Geometry: final body of the model. Coordinates: model frame, mm. Face numbers are marked on the shaded views. A direction names the side the tool comes from. Coordinates: 2 decimals unless noted, no trailing zeros. Loops run counter-clockwise (first coordinate to the right, second up) from the corner with the lowest first, then second, coordinate; pieces in that order, holes last. Notation, with made-up numbers: (-39.5, 54) - (12.5, 54) arc R21 ccw to (12.5, 80) - close; hole circle Ø6 at (42.25, 78). An arc over 180 degrees is marked (long way). Return JSON: item names as keys, results as strings.
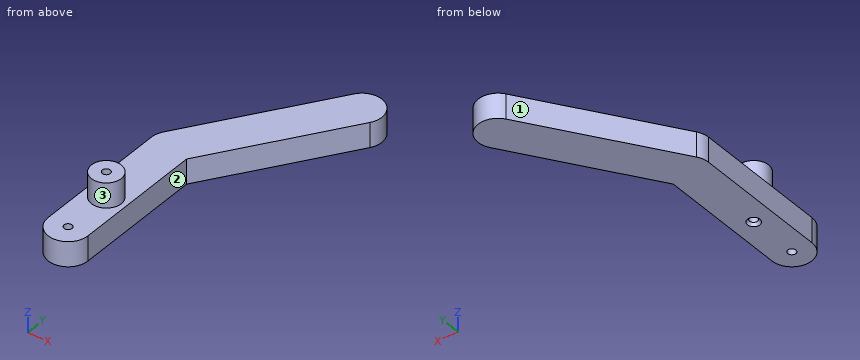
from build123d import *

# Parameters (mm, degrees)
F1_DEPTH       = 6.35
F2_R           = 3.81
F3_DEPTH       = 6.35
F4_D           = 2.032
F4_CSINK_D     = 3.175
F4_CSINK_ANGLE = 82
F5_D           = 2.032


with BuildPart() as f1:
    # F0 (on Top) → F1 (new body)
    with BuildSketch(Plane.XY):
        with BuildLine():
            ThreePointArc((-4.2115108686, 6.1978799769), (-0.9693096965, 8.3438461191), (2.8406999496, 7.5686908958))
            ThreePointArc((2.8406999496, 7.5686908958), (4.4853737717, 5.7420955662), (5.08, 3.3571800272))
            Line((5.08, 3.3571800272), (5.08, 1.8040681654))
            Line((5.08, 1.8040681654), (26.9371104656, 34.2085670262))
            ThreePointArc((26.9371104656, 34.2085670262), (25.5662995467, 41.2607778444), (18.5140887285, 39.8899669255))
            Line((18.5140887285, 39.8899669255), (-4.2115108686, 6.1978799769))
        make_face()
        with BuildLine():
            Line((0, 3.3571800272), (0, -1.7228199728))
            ThreePointArc((0, -1.7228199728), (2.384915539, -1.1281937445), (4.2115108686, 0.5164800776))
            Line((4.2115108686, 0.5164800776), (5.08, 1.8040681654))
            Line((5.08, 1.8040681654), (5.08, 3.3571800272))
            ThreePointArc((5.08, 3.3571800272), (4.4853737717, 5.7420955662), (2.8406999496, 7.5686908958))
            Line((2.8406999496, 7.5686908958), (0, 3.3571800272))
        make_face()
        with BuildLine():
            ThreePointArc((4.2115108686, 0.5164800776), (2.384915539, -1.1281937445), (0, -1.7228199728))
            ThreePointArc((0, -1.7228199728), (-3.5921024484, -0.2349224212), (-5.08, 3.3571800272))
            Line((-5.08, 3.3571800272), (-5.08, -30.9328199728))
            ThreePointArc((-5.08, -30.9328199728), (0, -36.0128199728), (5.08, -30.9328199728))
            Line((5.08, -30.9328199728), (5.08, 1.8040681654))
            Line((5.08, 1.8040681654), (4.2115108686, 0.5164800776))
        make_face()
        with BuildLine():
            ThreePointArc((-5.08, 3.3571800272), (-3.5921024484, -0.2349224212), (0, -1.7228199728))
            Line((0, -1.7228199728), (0, 3.3571800272))
            Line((0, 3.3571800272), (2.8406999496, 7.5686908958))
            ThreePointArc((2.8406999496, 7.5686908958), (-0.9693096965, 8.3438461191), (-4.2115108686, 6.1978799769))
            ThreePointArc((-4.2115108686, 6.1978799769), (-4.8580281603, 4.8424282872), (-5.08, 3.3571800272))
        make_face()
    extrude(amount=F1_DEPTH)

    # F2 (on face) → F3 (join)
    with BuildSketch(Plane.XY.offset(6.35)):
        with Locations((0, -18.2328199728)):
            Circle(F2_R)
    extrude(amount=F3_DEPTH)

    # F4 (through all)
    with Locations(Plane(origin=(0, 0, 0), x_dir=(1, 0, 0), z_dir=(0, 0, -1))):
        with Locations((0, 18.2328199728)):
            CounterSinkHole(F4_D / 2, F4_CSINK_D / 2, counter_sink_angle=F4_CSINK_ANGLE)

    # F5 (through all)
    with Locations(Plane(origin=(0, 0, 0), x_dir=(1, 0, 0), z_dir=(0, 0, -1))):
        with Locations((0, 30.9328199728)):
            Hole(F5_D / 2)


solid = f1.part
Item 1: Section query D-D, the plane z = 7.5. Return loops of the section in (x, y), and give its area (3 significant figures).
Worked out:
{"outline": "circle Ø7.62 at (0, -18.23); hole circle Ø2.03 at (0, -18.23)", "area": "42.4 mm^2"}
Item 2: Ray query, probe 1 along Y at (x, z) = (0, 5); probe 2 along X at (y, z) = (-23, 3.25); probe 3 along Z at (x, y) = (4, -15.5). Return the intervals inside material, ascending. Write a range as from..to.
Worked out:
{"probe 1": "-36.01..-31.95, -29.92..-19.25, -17.22..12.44", "probe 2": "-5.08..5.08", "probe 3": "0..6.35"}
Item 3: Section query B-B, the plane z = 1.5. Return loops of the section in (x, y).
Worked out:
{"outline": "(-5.08, -30.93) arc R5.08 ccw to (5.08, -30.93) - (5.08, 1.8) - (26.94, 34.21) arc R5.08 ccw to (18.51, 39.89) - (-4.21, 6.2) arc R5.08 ccw to (-5.08, 3.36) - close; hole circle Ø2.03 at (0, -30.93); hole circle Ø2.03 at (0, -18.23)"}
Item 4: Section query C-C, the plane y = -28.5. Return loops of the section in (x, z).
Worked out:
{"outline": "(-5.08, 0) - (5.08, 0) - (5.08, 6.35) - (-5.08, 6.35) - close"}
Item 5: Reachability of the marked faces 1, 2 and 3 from +Z, -Z, +X, -X, +Y, -Y: full face, straight path, thin tool, end or side. Return the list, or none.
Worked out:
{"face 1": "+Z, -Z, -X, +Y", "face 2": "+Z, -Z, +X, -Y", "face 3": "+Z"}
Item 6: Section query A-A, the plane x = 0. Return loops of the section in (y, z), and give its area (3 significant figures).
Worked out:
{"outline": "(-36.01, 0) - (-31.95, 0) - (-31.95, 6.35) - (-36.01, 6.35) - close; (-29.92, 0) - (-19.82, 0) - (-19.25, 0.66) - (-19.25, 12.7) - (-22.04, 12.7) - (-22.04, 6.35) - (-29.92, 6.35) - close; (-17.22, 0.66) - (-16.65, 0) - (12.44, 0) - (12.44, 6.35) - (-14.42, 6.35) - (-14.42, 12.7) - (-17.22, 12.7) - close", "area": "317 mm^2"}
Item 7: First-contact query: pin 1 Ø2.5 at (x, y) = (0, -30.93) entering from +Z; pin 2 Ø5 at (y, z) = (21.5, 8) entering from +X; pin 3 Ø1.8 at (x, y) = (0, -18.23) entering from +Z; pin 4 Ø4 at (x, z) = (1, 2.5) entering from +Y. Flat tips, straight axial feed; report the tip coordinate or a pass-through.
Worked out:
{"pin 1": "z = 6.35", "pin 2": "x = 19.63", "pin 3": "through", "pin 4": "y = 16.89"}
